Print and shaded views of the part. All mm, measured from the part's lowest x, y and z. A direction names the side the tool comes from. Round coordinates to 2 decimals unless told otherwise and drop trailing zeros. Loops run counter-clockwise (first coordinate to the right, second up) from the corner with the lowest first, then second, coordinate; pieces in that order, holes last. Notation, with made-up numbers: (63, 64.25) - (67, 64.25) arc R18 ccw to (67, 83.25) - close; hole circle Ø9 at (71.25, -10.75). An arc over 180 degrees is marked (long way). Use one line per item in the form item = value. Start each with the question number.
Q1. Pin check, flat tips, straight feed: pin 1 (2.5 mm diameter, centred on y = 4, z = 3.5, fed in from +X); pin 2 (5 mm diameter, centred on x = 64.5, y = 4.5, fed in from +Z); pin 3 (5.5 mm diameter, centred on y = 6.5, z = 2, fed in from -X). Stop position of each tip, or through.
Q2. Saw through at A-A (z = 4). Give the cut face in (x, y), then the cut area to 3 significant figures.
Q3. Saw through at B-B (y = 2). Give the cut face in (x, z), then the cut area to 3 significant figures.
Q4. Saw through at C-C (x = 66). Give the cut face in (y, z), then the cut area to 3 significant figures.
Q5. Mould opens along X. For the marked faces 1, 2 and 3 say: released by +X, released by -X, zero draft, split by the parting line, or undercut.
Q6. Drill centre line: line 1 (Z direction, x = 7, y = 0.75). Where is it in solid material? Low to high.
Q7. 3-axis set-ups, long thin cutter, end or side, ignore diameter. For the marked faces 4, 5, 6, 7 and 8: which of +Z, -Z, +X, -X, +Y, -Y reach the whole face in a straight line?
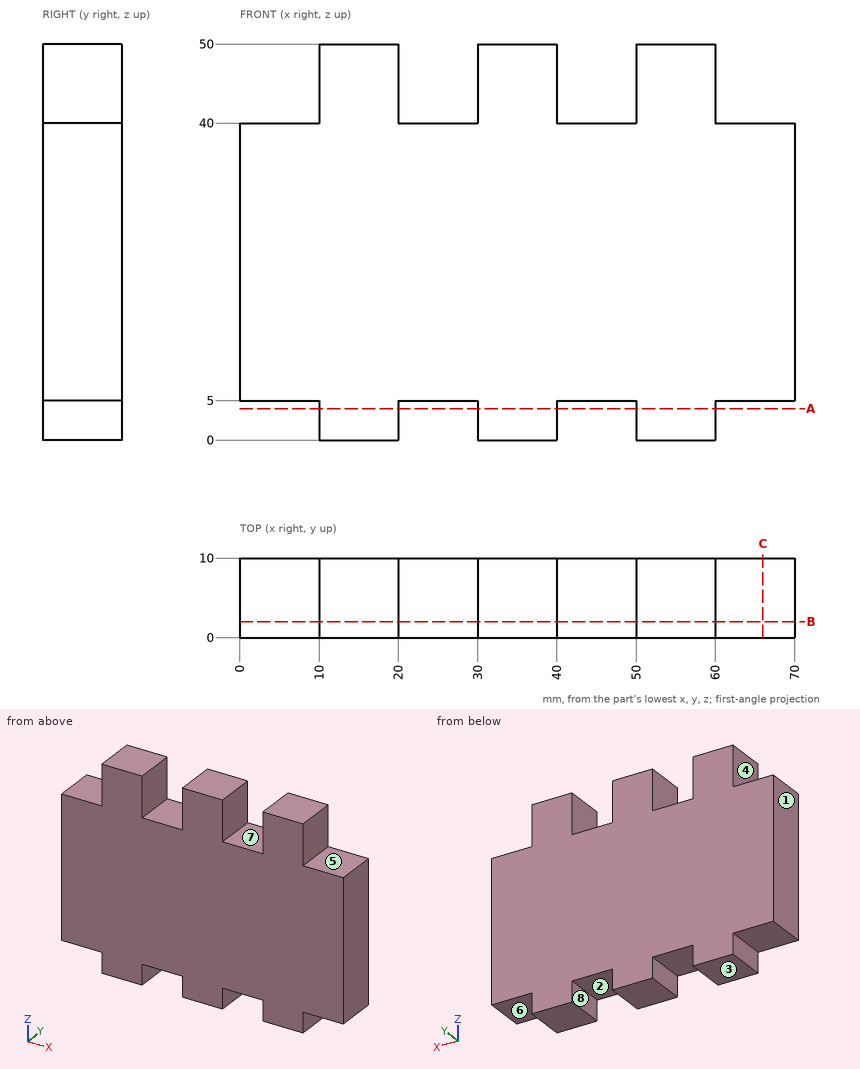
Report:
q1.pin_1 = 60
q1.pin_2 = 40
q1.pin_3 = 10
q2.outline = (10, 0) - (20, 0) - (20, 10) - (10, 10) - close; (30, 0) - (40, 0) - (40, 10) - (30, 10) - close; (50, 0) - (60, 0) - (60, 10) - (50, 10) - close
q2.area = 300 mm²
q3.outline = (0, 5) - (10, 5) - (10, 0) - (20, 0) - (20, 5) - (30, 5) - (30, 0) - (40, 0) - (40, 5) - (50, 5) - (50, 0) - (60, 0) - (60, 5) - (70, 5) - (70, 40) - (60, 40) - (60, 50) - (50, 50) - (50, 40) - (40, 40) - (40, 50) - (30, 50) - (30, 40) - (20, 40) - (20, 50) - (10, 50) - (10, 40) - (0, 40) - close
q3.area = 2,900 mm²
q4.outline = (0, 5) - (10, 5) - (10, 40) - (0, 40) - close
q4.area = 350 mm²
q5.face_1 = released by -X
q5.face_2 = undercut
q5.face_3 = zero draft
q6.line_1 = 5 to 40
q7.face_4 = +Z, -X, +Y, -Y
q7.face_5 = +Z, +X, +Y, -Y
q7.face_6 = -Z, +X, +Y, -Y
q7.face_7 = +Z, +Y, -Y
q7.face_8 = -Z, +Y, -Y
